Can you work these out from the model? Positions are in its coordinate system, mm. A direction names the side the tool comes from. Round coordinates to 2 decimals unless told otherwise and drop trailing zeros. Order: outer loops, then holes, each group sorted by start corner. A loop starts at its lowest first (then second) coordinate and runs counter-clockwise, first axis right, second up. Notation, with made-up numbers: (-28, 88.25) - (29, 88.25) arc R26 ccw to (29, 115.25) - close; hole circle Ø1 at (9.25, 61). An arc over 180 degrees is marked (long way). Write item = value, one per line.
Autodesk Inventor part; units mm, degrees
ref_plane "YZ Plane" through (0, 0, 0) normal (1, 0, 0) x (0, 1, 0)
ref_plane "XZ Plane" through (0, 0, 0) normal (0, 1, 0) x (-1, 0, 0)
ref_plane "XY Plane" through (0, 0, 0) normal (0, 0, 1) x (1, 0, 0)
sketch "Sketch1" plane through (0, 0, 0) normal (1, 0, 0) x (0, 1, 0)
  line L0 (0, 0) -> (16.383, 0)
  line L1 (16.383, 0) -> (16.383, -15.875)
  line L2 (16.383, -15.875) -> (0, -15.875)
  line L3 (0, -15.875) -> (0, 0)
  dimension "d0" = 16.383
  dimension "d1" = 15.875
extrude "Extrusion1" add sketch "Sketch1" along normal blind 184.15
sketch "Sketch2" plane through (0, 0, -15.875) normal (0, 0, -1) x (-1, 0, 0)
  line L0 (-184.15, 16.383) -> (-184.15, 0)
  line L1 (-184.15, 16.383) -> (-176.53, 16.383)
  line L2 (0, 16.383) -> (-184.15, 16.383)
  line L3 (-176.53, 16.383) -> (-176.53, 13.081)
  line L4 (-176.53, 13.081) -> (-181.61, 13.081)
  line L5 (-181.61, 13.081) -> (-181.61, 8.001)
  line L6 (-181.61, 8.001) -> (-176.53, 8.001)
  line L7 (-176.53, 8.001) -> (-176.53, 2.921)
  line L8 (-176.53, 2.921) -> (-171.45, 2.921)
  line L9 (-171.45, 2.921) -> (-171.45, 8.001)
  line L10 (-171.45, 8.001) -> (-166.37, 8.001)
  line L11 (-166.37, 8.001) -> (-166.37, 13.081)
  line L12 (-166.37, 13.081) -> (-171.45, 13.081)
  line L13 (-171.45, 16.383) -> (-171.45, 13.081)
  line L14 (0, 16.383) -> (-7.62, 16.383)
  line L15 (-7.62, 16.383) -> (-7.62, 13.081)
  line L16 (-7.62, 13.081) -> (-2.54, 13.081)
  line L17 (-2.54, 13.081) -> (-2.54, 8.001)
  line L18 (-2.54, 8.001) -> (-7.62, 8.001)
  line L19 (-7.62, 8.001) -> (-7.62, 2.921)
  line L20 (-7.62, 2.921) -> (-12.7, 2.921)
  line L21 (-12.7, 2.921) -> (-12.7, 8.001)
  line L22 (-12.7, 8.001) -> (-17.78, 8.001)
  line L23 (-17.78, 8.001) -> (-17.78, 13.081)
  line L24 (-17.78, 13.081) -> (-12.7, 13.081)
  line L25 (-12.7, 13.081) -> (-12.7, 16.383)
  point P0 (0, 0)
  dimension "d4" = 7.62
  dimension "d5" = 3.302
  dimension "d6" = 5.08
  dimension "d7" = 5.08
  dimension "d8" = 5.08
  dimension "d9" = 5.08
  dimension "d10" = 5.08
  dimension "d11" = 7.62
  dimension "d12" = 3.302
  dimension "d13" = 5.08
  dimension "d14" = 5.08
  dimension "d15" = 5.08
extrude "Extrusion2" cut sketch "Sketch2" against normal blind 184.15
shell "Shell1" thickness 1.778 removed faces 0
properties part number "horzntalconnection"
(1) If we section it at B-B (x = 98): Write out the boundary of the cut face in (y, z) (3 decimals), plus the area to 3 significant figures.
Computed:
outline = (0, -15.875) - (16.383, -15.875) - (16.383, 0) - (0, 0) - close; hole (1.778, -14.097) - (14.605, -14.097) - (14.605, -1.778) - (1.778, -1.778) - close
area = 102 mm^2
(2) Thinking about a two-plate mould opening in X: for faces 1 (the face through (91, 0, -8)), 2 (the face through (167, 6.223, -8)), 3 (the face through (4, 4, -14.097)), which applies, +X half, -X half, draft (parallel to the pull), parting line (faces both ways), or undercut?
Computed:
face_1 = draft
face_2 = undercut
face_3 = undercut
(3) If we section it at A-A (y = 4.5): Write out the boundary of the cut face in (x, z) (3 decimals), plus the area to 3 significant figures.
Computed:
outline = (0, -15.875) - (7.62, -15.875) - (7.62, 0) - (0, 0) - close; (12.7, -15.875) - (171.45, -15.875) - (171.45, 0) - (12.7, 0) - close; (176.53, -15.875) - (184.15, -15.875) - (184.15, 0) - (176.53, 0) - close; hole (1.778, -14.097) - (5.842, -14.097) - (5.842, -1.778) - (1.778, -1.778) - close; hole (14.478, -14.097) - (169.672, -14.097) - (169.672, -1.778) - (14.478, -1.778) - close; hole (178.308, -14.097) - (182.372, -14.097) - (182.372, -1.778) - (178.308, -1.778) - close
area = 750 mm^2
(4) On a 3-axis mill with a long thin cutter (end or side, diameter ignored), from which of +Z, -Z, +X, -X, +Y, -Y can I reach the whole of each face in a straight line? I mean faces 4 (the face through (174, 2.921, -8)), 5 (the face through (2.54, 11, -8)), 6 (the face through (4, 4, -1.778)). Say none if no direction works.
Computed:
face_4 = +Z, -Z, +Y
face_5 = +Z, -Z
face_6 = none
(5) If I drill on line 1 (X direction, y = 8.75, z = -4.75); line 2 (X direction, y = 3, z = -12); line 3 (X direction, y = 8.75, z = -14.25), over which ranges is the centre line in solid material (lowest first)? Write a range as from..to.
Computed:
line_1 = 0..2.54, 17.78..19.56, 164.59..166.37, 181.61..184.15
line_2 = 0..1.78, 5.84..7.62, 12.7..14.48, 169.67..171.45, 176.53..178.31, 182.37..184.15
line_3 = 0..2.54, 17.78..166.37, 181.61..184.15
(6) If we section it at C-C (z = -4.75): State how many separate pieces and enclosed holes the cut face has, plus the area to 3 significant figures.
Computed:
separate_pieces = 1
enclosed_holes = 3
area = 835 mm^2
